Verification items for the finished model (mm, model axes). Face numbers are marked on the shaded views. A direction names the side the tool comes from. Give positions to 0.01 mm unless a question says otherwise; leave off trailing zeros. Order: outer loops, then holes, each group sorted by start corner. A loop starts at its lowest first (then second) coordinate and runs counter-clockwise, first axis right, second up.
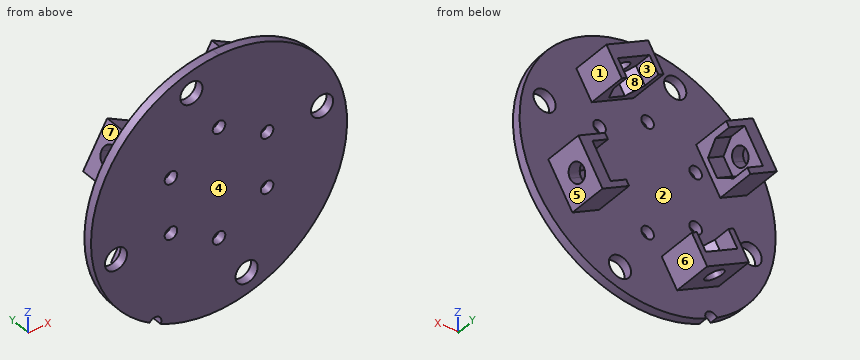
from build123d import *

# Parameters (mm, degrees)
SKETCH1_R           = 30
SKETCH1_R_2         = 1.475
SKETCH1_R_3         = 2.6
BOSS_EXTRUDE1_DEPTH = 2
SKETCH2_R           = 1.5
CUT_EXTRUDE1_DEPTH  = 10
BOSS_EXTRUDE3_DEPTH = 9.1
CIRPATTERN1_COUNT   = 4
CUT_EXTRUDE2_START  = -3
CUT_EXTRUDE2_DEPTH  = 5
CUT_EXTRUDE3_DEPTH  = 15
CIRPATTERN2_COUNT   = 4
CIRPATTERN3_COUNT   = 4


with BuildPart() as part:
    # Sketch1 → Boss-Extrude1 (new body)
    with BuildSketch(Plane(origin=(0, 0, 0), x_dir=(1, 0, 0), z_dir=(0, 1, 0))):
        with Locations(Location((0, 0, 0), (0, 0, 270))):
            Circle(SKETCH1_R)
        with Locations(Location((0, 13, 0), (0, 0, 270))):
            Circle(SKETCH1_R_2, mode=Mode.SUBTRACT)
        with Locations(Location((11.258330249, 6.5, 0), (0, 0, 270))):
            Circle(SKETCH1_R_2, mode=Mode.SUBTRACT)
        with Locations(Location((11.258330249, -6.5, 0), (0, 0, 270))):
            Circle(SKETCH1_R_2, mode=Mode.SUBTRACT)
        with Locations(Location((0, -13, 0), (0, 0, 270))):
            Circle(SKETCH1_R_2, mode=Mode.SUBTRACT)
        with Locations(Location((-11.258330249, -6.5, 0), (0, 0, 270))):
            Circle(SKETCH1_R_2, mode=Mode.SUBTRACT)
        with Locations(Location((-11.258330249, 6.5, 0), (0, 0, 270))):
            Circle(SKETCH1_R_2, mode=Mode.SUBTRACT)
        with Locations(Location((-24.148145657, 6.470476128, 0), (0, 0, 270))):
            Circle(SKETCH1_R_3, mode=Mode.SUBTRACT)
        with Locations(Location((6.470476128, 24.148145657, 0), (0, 0, 270))):
            Circle(SKETCH1_R_3, mode=Mode.SUBTRACT)
        with Locations(Location((24.148145657, -6.470476128, 0), (0, 0, 270))):
            Circle(SKETCH1_R_3, mode=Mode.SUBTRACT)
        with Locations(Location((-6.470476128, -24.148145657, 0), (0, 0, 270))):
            Circle(SKETCH1_R_3, mode=Mode.SUBTRACT)
    extrude(amount=BOSS_EXTRUDE1_DEPTH)

    # Sketch2 → Cut-Extrude1 (cut)
    with BuildSketch(Plane(origin=(0, 2, 0), x_dir=(1, 0, 0), z_dir=(0, 1, 0))):
        with Locations((-15, 25.980762114)):
            Circle(SKETCH2_R)
    extrude(amount=-CUT_EXTRUDE1_DEPTH, mode=Mode.SUBTRACT)

    # Sketch8 → Boss-Extrude3 (add)
    with BuildSketch(Plane(origin=(0, 2, 0), x_dir=(1, 0, 0), z_dir=(0, 1, 0))):
        Polygon((-6.906956469, 23.263199529), (-11.8, 20.438199529), (-8.2, 14.202816622), (-3.306956469, 17.027816622), align=None)
        Polygon((-8.2, 14.202816622), (-11.8, 20.438199529), (-16.693043531, 17.613199529), (-13.093043531, 11.377816622), align=None)
    boss_extrude3 = extrude(amount=BOSS_EXTRUDE3_DEPTH)

    # CirPattern1: Boss-Extrude3 ×4 about axis
    cirpattern1_axis = Axis((0, 0, 0), (0, 1, 0))
    for i in range(1, CIRPATTERN1_COUNT):
        add(boss_extrude3.rotate(cirpattern1_axis, i * 360 / CIRPATTERN1_COUNT))

    # Sketch9 → Cut-Extrude2 (cut)
    with BuildSketch(Plane(origin=(-11.8, 0, -20.438199529), x_dir=(-0.8660254037844384, 0, 0.5000000000000006), z_dir=(-0.5000000000000006, 0, -0.8660254037844384)).offset(CUT_EXTRUDE2_START)):
        Polygon((0, 3.3), (0, 10.7), (-2.136195996, 10.7), (-4.272391992, 7), (-2.136195996, 3.3), align=None)
        Polygon((2.136195996, 10.7), (0, 10.7), (0, 3.3), (2.136195996, 3.3), (4.272391992, 7), align=None)
        Polygon((0, 10.7), (0, 11.1), (-4.272391992, 11.1), (-4.272391992, 7), (-2.136195996, 10.7), align=None)
        Polygon((4.272391992, 11.1), (0, 11.1), (0, 10.7), (2.136195996, 10.7), (4.272391992, 7), align=None)
    cut_extrude2 = extrude(amount=-CUT_EXTRUDE2_DEPTH, mode=Mode.SUBTRACT)

    # Sketch10 → Cut-Extrude3 (cut)
    with BuildSketch(Plane(origin=(-11.8, 0, -20.438199529), x_dir=(-0.8660254037844384, 0, 0.5000000000000006), z_dir=(-0.5000000000000006, 0, -0.8660254037844384))):
        with BuildLine():
            ThreePointArc((2.1, 7), (1.48492424, 8.48492424), (0, 9.1))
            Line((0, 9.1), (0, 4.9))
            ThreePointArc((0, 4.9), (1.48492424, 5.51507576), (2.1, 7))
        make_face()
        with BuildLine():
            Line((0, 4.9), (0, 9.1))
            ThreePointArc((0, 9.1), (-2.1, 7), (0, 4.9))
        make_face()
    cut_extrude3 = extrude(amount=-CUT_EXTRUDE3_DEPTH, mode=Mode.SUBTRACT)

    # CirPattern2: Cut-Extrude2 ×4 about axis
    cirpattern2_axis = Axis((0, 0, 0), (0, 1, 0))
    for i in range(1, CIRPATTERN2_COUNT):
        add(cut_extrude2.rotate(cirpattern2_axis, i * 360 / CIRPATTERN2_COUNT), mode=Mode.SUBTRACT)

    # CirPattern3: Cut-Extrude3 ×4 about axis
    cirpattern3_axis = Axis((0, 2, 0), (0, 1, 0))
    for i in range(1, CIRPATTERN3_COUNT):
        add(cut_extrude3.rotate(cirpattern3_axis, i * 360 / CIRPATTERN3_COUNT), mode=Mode.SUBTRACT)


solid = part.part
(1) Go/stop test with flat-tipped pins: pin 1 (1.7 mm diameter, centred on x = 9.5, z = 15, fed in from +Y); pin 2 (4 mm diameter, centred on x = 7, y = 3, fed in from -Z); pin 3 (4 mm diameter, centred on y = 8.5, z = 10, fed in from +X). Record where each tip stops, or that it passes through.
Solved:
pin 1: stops at y = 3.3
pin 2: stops at z = -29.53
pin 3: stops at x = 13.45
(2) Section check A-A, the plane y = 10.25. Give the number of separate pieces and of enclosed holes in the cut face, then the cut area to 3 significant figures.
Solved:
separate pieces: 4
enclosed holes: 0
area: 182 mm2
(3) Section check C-C, the plane z = 0. Enter the section's corners in (x, y), then the cut area to 3 significant figures.
Solved:
outline: (-30, 0) - (30, 0) - (30, 2) - (-30, 2) - close
area: 120 mm2
(4) Release check for a two-part mould opening along X. For the marked faces 6, 7 and 8 record: pulls with the +X half, pulls with the -X half, needs draft (parallel to the pull), parting line crosses it, or undercut.
Solved:
face 6: pulls with the +X half
face 7: pulls with the -X half
face 8: undercut
(5) Scan lines: line 1 (X direction, y = 10, z = -12.5); line 2 (X direction, y = 0.9, z = -6.5); line 3 (X direction, y = 9, z = 12.5). Record each from-to range of solid material in increasing order.
Solved:
line 1: x = -13.74 to -12.15, 11.72 to 13.11, 16.57 to 20.03
line 2: x = -29.29 to -26.75, -21.55 to -12.73, -9.78 to 9.78, 12.73 to 29.29
line 3: x = -20.03 to -16.57, -13.11 to -11.72, 12.15 to 13.74
(6) Set-up check for the marked faces 1, 2, 3, 4 and 5: record each of +Z, -Z, +X, -X, +Y, -Y from which the full face is reachable in a straight line by a thin tool's end or side.
Solved:
face 1: +X, +Y
face 2: +Y
face 3: -Z, +Y
face 4: +Z, -Z, +X, -X, -Y
face 5: -Z, +X, +Y
